Build history of the part. All positions in model axes, mm. Face numbers are marked on the shaded views. Round coordinates to 2 decimals unless told otherwise and drop trailing zeros. Write each loop counter-clockwise with the first axis right and the second up, starting at its lowest first coordinate (ties: lowest second). Pieces come first, ordered by that corner, then holes.
Item 1: Band-saw the part on B-B, the plane z = -133. Write the cut outline in (x, y).
Item 2: Mould opens along Z. For the marked faces 1 and 2 say: +Z half, -Z half, draft (parallel to the pull), parting line (faces both ways), or undercut.
Item 3: Drop flat-ended pins along their axis: pin 1 Ø1 at (y, z) = (1, -122) entering from -X; pin 2 Ø2.5 at (x, z) = (15, -143.7) entering from -Y. Give the stop position or say it passes through.
Item 4: Wall check: probe 1 along Z at (x, y) = (222, 4.5); probe 2 along X at (y, z) = (6.25, -26.5); probe 3 along Z at (x, y) = (227.8, 1). Give the ranges that are in metal, low to high.
Item 5: Band-saw the part on A-A, the plane x = 37. Write the cut outline in (y, z).
```python
from build123d import *

# Parameters (mm, degrees)
SKIZZE1_W                          = 242.8
SKIZZE1_H                          = 158.7
AUFSATZ_LINEAR_AUSTRAGEN1_DEPTH    = 7.5
VERRUNDUNG1_R                      = 10
WANDUNG1_T                         = -2
F_3_0_3_DURCHMESSER_BOHRUNG1_D     = 3
F_3_0_3_DURCHMESSER_BOHRUNG1_DEPTH = 6
F_3_0_3_DURCHMESSER_BOHRUNG1_TIP   = 0.901290929
SKIZZE5_W                          = 204.8
SKIZZE5_H                          = 120.7
SCHNITT_LINEAR_AUSTRAGEN1_DEPTH    = 291.116838532
VERRUNDUNG2_R                      = 2
SKIZZE6_W                          = 17
SKIZZE6_H                          = 36.7
SCHNITT_LINEAR_AUSTRAGEN2_DEPTH    = 7.5
AUFSATZ_LINEAR_START               = -2
SKIZZE8_W                          = 52
SKIZZE8_H                          = 4
AUFSATZ_LINEAR_AUSTRAGEN2_DEPTH    = 7.5


with BuildPart() as part:
    # Skizze1 → Aufsatz-Linear austragen1 (new body)
    with BuildSketch(Plane(origin=(0, 0, 0), x_dir=(1, 0, 0), z_dir=(0, 1, 0))):
        with Locations((121.4, 79.35)):
            Rectangle(SKIZZE1_W, SKIZZE1_H)
    extrude(amount=AUFSATZ_LINEAR_AUSTRAGEN1_DEPTH)

    # Verrundung1
    verrundung1_edges = [part.edges().sort_by_distance(p)[0] for p in [
        (0, 3.75, -158.7),
        (242.8, 3.75, -158.7),
        (242.8, 3.75, 0),
        (0, 3.75, 0),
    ]]
    fillet(verrundung1_edges, radius=VERRUNDUNG1_R)

    # Wandung1
    wandung1_openings = [part.faces().sort_by_distance(p)[0] for p in [
        (121.4, 7.5, -79.35),
    ]]
    offset(amount=WANDUNG1_T, openings=wandung1_openings, kind=Kind.INTERSECTION)

    # Ø3.0 (3) Durchmesser Bohrung1
    with Locations(Plane(origin=(0, 2, 0), x_dir=(1, 0, 0), z_dir=(0, 1, 0))):
        with Locations((15, 143.7), (105, 143.7), (227.8, 143.7), (227.8, 15), (105, 15), (15, 15)):
            Hole(F_3_0_3_DURCHMESSER_BOHRUNG1_D / 2, depth=F_3_0_3_DURCHMESSER_BOHRUNG1_DEPTH)
            with Locations((0, 0, -(F_3_0_3_DURCHMESSER_BOHRUNG1_DEPTH + F_3_0_3_DURCHMESSER_BOHRUNG1_TIP / 2))):  # 118° drill point
                Cone(0, F_3_0_3_DURCHMESSER_BOHRUNG1_D / 2, F_3_0_3_DURCHMESSER_BOHRUNG1_TIP, mode=Mode.SUBTRACT)

    # Skizze5 → Schnitt-Linear austragen1 (cut, through all)
    with BuildSketch(Plane(origin=(0, 2, 0), x_dir=(1, 0, 0), z_dir=(0, 1, 0))):
        with Locations((121.4, 79.35)):
            Rectangle(SKIZZE5_W, SKIZZE5_H)
    extrude(amount=-SCHNITT_LINEAR_AUSTRAGEN1_DEPTH, mode=Mode.SUBTRACT)

    # Verrundung2
    verrundung2_edges = [part.edges().sort_by_distance(p)[0] for p in [
        (0, 0, -79.35),
        (121.4, 0, -158.7),
        (242.8, 0, -79.35),
        (121.4, 0, 0),
        (239.871067812, 0, -2.928932188),
        (2.928932188, 0, -2.928932188),
        (239.871067812, 0, -155.771067812),
        (2.928932188, 0, -155.771067812),
    ]]
    fillet(verrundung2_edges, radius=VERRUNDUNG2_R)

    # Skizze6 → Schnitt-Linear austragen2 (cut)
    with BuildSketch(Plane.XZ):
        with Locations((232.3, -88.35)):
            Rectangle(SKIZZE6_W, SKIZZE6_H)
    extrude(amount=-SCHNITT_LINEAR_AUSTRAGEN2_DEPTH, mode=Mode.SUBTRACT)

    # Skizze8 → Aufsatz-Linear austragen2 (add)
    with BuildSketch(Plane(origin=(0, 2, 0), x_dir=(1, 0, 0), z_dir=(0, 1, 0)).offset(AUFSATZ_LINEAR_START)):
        with Locations((214.8, 108.7)):
            Rectangle(SKIZZE8_W, SKIZZE8_H)
        with Locations((214.8, 68)):
            Rectangle(SKIZZE8_W, SKIZZE8_H)
    extrude(amount=AUFSATZ_LINEAR_AUSTRAGEN2_DEPTH)


solid = part.part
```
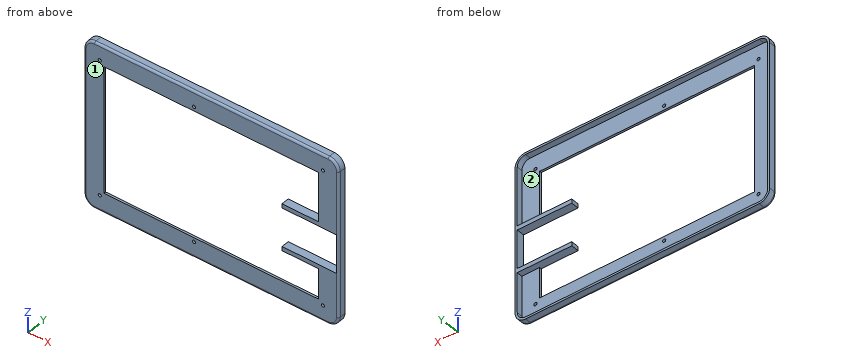
Results:
1. outline: (0, 2) arc R2 ccw to (2, 0) - (19, 0) - (19, 2) - (2, 2) - (2, 7.5) - (0, 7.5) - close; (223.8, 0) - (240.8, 0) arc R2 ccw to (242.8, 2) - (242.8, 7.5) - (240.8, 7.5) - (240.8, 2) - (223.8, 2) - close
2. face 1: draft
2. face 2: undercut
3. pin 1: stops at x = 0.06
3. pin 2: passes through
4. probe 1: z = -158.7 to -156.7, -110.7 to -106.7, -70 to -66, -2 to 0
4. probe 2: x = 0 to 2, 240.8 to 242.8
4. probe 3: z = -158.43 to -145.2, -142.2 to -106.7, -70 to -16.5, -13.5 to -0.27
5. outline: (0, -156.7) arc R2 ccw to (2, -158.7) - (7.5, -158.7) - (7.5, -156.7) - (2, -156.7) - (2, -139.7) - (0, -139.7) - close; (0, -19) - (2, -19) - (2, -2) - (7.5, -2) - (7.5, 0) - (2, 0) arc R2 ccw to (0, -2) - close
